Autodesk Inventor part; units mm, degrees
ref_plane "YZ Plane" through (0, 0, 0) normal (1, 0, 0) x (0, 1, 0)
ref_plane "XZ Plane" through (0, 0, 0) normal (0, 1, 0) x (-1, 0, 0)
ref_plane "XY Plane" through (0, 0, 0) normal (0, 0, 1) x (1, 0, 0)
sketch "Sketch1" plane through (0, 0, 0) normal (0, 0, 1) x (1, 0, 0)
  circle A0 centre (0, 0) radius 16.5
  circle A1 centre (-47.5262, 0) radius 20
  circle A2 centre (0, 0) radius 73
  circle A3 centre (-23.7631, -41.1589) radius 20
  circle A4 centre (23.7631, -41.1589) radius 20
  circle A5 centre (47.5262, 0) radius 20
  circle A6 centre (23.7631, 41.1589) radius 20
  circle A7 centre (-23.7631, 41.1589) radius 20
  point P0 (0, 66.675)
  point P1 (-57.7422, 33.3375)
  point P2 (-57.7422, -33.3375)
  point P3 (0, -66.675)
  point P4 (57.7422, -33.3375)
  point P5 (57.7422, 33.3375)
  point P6 (0, 22)
  point P7 (-19.0526, 11)
  point P8 (-19.0526, -11)
  point P9 (0, -22)
  point P10 (19.0526, -11)
  point P11 (19.0526, 11)
  dimension "d0" = 66.675
  dimension "d3" = 360
  dimension "d9" = 33
  dimension "d19" = 40
  dimension "d20" = 22
  dimension "d23" = 360
  dimension "d25" = 146
  dimension "d28" = 360
extrude "Extrusion2" add sketch "Sketch1" along normal blind 6
hole "Hole2" at (0, 66.675, 0) at (-57.7422, 33.3375, 0) at (-57.7422, -33.3375, 0) at (0, -66.675, 0) at (57.7422, -33.3375, 0) at (57.7422, 33.3375, 0) direction (0, 0, 1) diameter 6.5 end through all
hole "Hole3" at (0, 22, 0) at (-19.0526, 11, 0) at (-19.0526, -11, 0) at (0, -22, 0) at (19.0526, 11, 0) at (19.0526, -11, 0) direction (0, 0, 1) diameter 5 end through all
properties part number "SprocketHubPlate"
Input: part model. Units: mm. Frame: model coordinates. Coordinates: 2 decimals unless noted, no trailing zeros. Loops run counter-clockwise (first coordinate to the right, second up) from the corner with the lowest first, then second, coordinate; pieces in that order, holes last.
Q1. Mould query, pull axis X, two halves, no side actions, for faces 1 (the flat face through (15, -15, 0)), 2 (the cylindrical face through (59.72, -35.917, 3.042)), 3 (the cylindrical face through (-15.825, 71.264, 2.958)). Classes: +X half, -X half, draft (parallel to the pull), parting line (faces both ways), or undercut.
Results are:
face 1: draft
face 2: undercut
face 3: parting line
Q2. Line query: line 1 along Y through (x, z) = (0, 3.75) (3 decimals); line 2 along Y through (x, z) = (-25, 1.55); line 3 along X through (y, z) = (-55, 4.75). Output: solid intervals per line, ascending.
Results are:
line 1: y = -73 to -69.925, -63.425 to -24.5, -19.5 to -16.5, 16.5 to 19.5, 24.5 to 63.425, 69.925 to 73
line 2: y = -68.59 to -61.12, -21.2 to 21.2, 61.12 to 68.59
line 3: x = -48 to -38.2, -9.33 to 9.33, 38.2 to 48
Q3. Section D-D, the plane x = 48.5. Return the cut outline in (y, z), and give its area (3 significant figures).
Results are:
outline: (-54.56, 0) - (-19.98, 0) - (-19.98, 6) - (-54.56, 6) - close; (19.98, 0) - (54.56, 0) - (54.56, 6) - (19.98, 6) - close
area: 415 mm2
Q4. Section A-A, the plane x = 0. Return the cut outline in (y, z) (3 decimals), and give its area (3 significant figures).
Results are:
outline: (-73, 0) - (-69.925, 0) - (-69.925, 6) - (-73, 6) - close; (-63.425, 0) - (-24.5, 0) - (-24.5, 6) - (-63.425, 6) - close; (-19.5, 0) - (-16.5, 0) - (-16.5, 6) - (-19.5, 6) - close; (16.5, 0) - (19.5, 0) - (19.5, 6) - (16.5, 6) - close; (24.5, 0) - (63.425, 0) - (63.425, 6) - (24.5, 6) - close; (69.925, 0) - (73, 0) - (73, 6) - (69.925, 6) - close
area: 540 mm2
Q5. Section C-C, the plane z = 1.85. Give the number of separate pieces and of enclosed holes in the cut face, and give its area (3 significant figures).
Results are:
separate pieces: 1
enclosed holes: 19
area: 8,030 mm2
Q6. Contact query for flat-ended pins moving along their axis: pin 1 (4 mm diameter, centred on x = 0, y = -22, fed in from +Z); pin 2 (2 mm diameter, centred on x = 43, z = 4, fed in from +Y); pin 3 (1.5 mm diameter, centred on y = -36.5, z = 2, fed in from -X); pin 4 (6 mm diameter, centred on x = -2, y = 26.5, fed in from -Z). Output: stop coordinate, or through.
Results are:
pin 1: passes through
pin 2: stops at y = 59.71
pin 3: stops at x = -63.65
pin 4: stops at z = 0
Q7. Section B-B, the plane y = -11. Return the cut outline in (x, z), and give its area (3 significant figures).
Results are:
outline: (-72.17, 0) - (-64.23, 0) - (-64.23, 6) - (-72.17, 6) - close; (-30.82, 0) - (-21.55, 0) - (-21.55, 6) - (-30.82, 6) - close; (-16.55, 0) - (-12.3, 0) - (-12.3, 6) - (-16.55, 6) - close; (12.3, 0) - (16.55, 0) - (16.55, 6) - (12.3, 6) - close; (21.55, 0) - (30.82, 0) - (30.82, 6) - (21.55, 6) - close; (64.23, 0) - (72.17, 0) - (72.17, 6) - (64.23, 6) - close
area: 258 mm2
